Part model, mm, in its own coordinate system. Coordinates: 2 decimals unless noted, no trailing zeros. Write each loop counter-clockwise with the first axis right and the second up, starting at its lowest first coordinate (ties: lowest second). Pieces come first, ordered by that corner, then holes. Notation, with made-up numbers: (-40, 41.25) -> (-25, 41.25) arc R11 cw to (-25, 57.25) -> close; hole circle Ø4 at (59, -39). An arc over 180 degrees is marked (long way). One line per question, with ' | ' between items. Start each with the question number.
Item 1: Saw through at D-D (x = 0). List the corners of the cut face in (y, z), and give its area (3 significant figures).
Item 2: Two-plate mould, pull along Y, no slides. Class faces 1 (the cylindrical face through (-1.5, -4.5, -3.5)), 2 (the flat face through (-2, 0, -6)), 3 (the cylindrical face through (1.5, -4.5, -3.5)), 4 (the cylindrical face through (0.028, -5.158, -3.955)): pulls with the +Y half, pulls with the -Y half, needs draft (parallel to the pull), parting line crosses it, or undercut.
Item 3: Pin check, flat tips, straight feed: pin 1 (2 mm diameter, centred on x = 1.5, z = -3, fed in from -Y); pin 2 (3 mm diameter, centred on y = 0, z = 0, fed in from +X); pin 3 (2 mm diameter, centred on x = 1.5, y = -4, fed in from +Z); pin 4 (1 mm diameter, centred on x = -1.5, y = 3, fed in from +Z). Stop position of each tip, or through.
Item 4: Probe probe 1 along Z at (x, y) = (-1.65, 0); probe 2 along Z at (x, y) = (0.2, 0); probe 3 along Y at (x, z) = (1.45, -1.25). List the from-to ranges inside material, lowest first. Write a range as [from, to].
Item 5: Saw through at A-A (z = 0). List the corners of the cut face in (x, y).
Item 6: Saw through at C-C (x = 1.4). List the corners of the cut face in (y, z).
from build123d import *


with BuildPart() as part:
    # Esquisse1 → Révolution1 (revolve)
    with BuildSketch(Plane.XY):
        with BuildLine():
            Line((-2, 6.5), (2, 6.5))
            Line((2, 6.5), (2, 5.7))
            Line((2, 5.7), (1.058300524, 5.7))
            ThreePointArc((1.058300524, 5.7), (1.6, 4.5), (1.058300524, 3.3))
            Line((1.058300524, 3.3), (2, 3.3))
            Line((2, 3.3), (2, 2.5))
            Line((2, 2.5), (-2, 2.5))
            Line((-2, 2.5), (-2, 3.3))
            Line((-2, 3.3), (-1.058300524, 3.3))
            ThreePointArc((-1.058300524, 3.3), (-1.6, 4.5), (-1.058300524, 5.7))
            Line((-1.058300524, 5.7), (-2, 5.7))
            Line((-2, 5.7), (-2, 6.5))
        make_face()
    revolve(axis=Axis((-3.50151098, 0, 0), (1, 0, 0)))


solid = part.part
From the geometry:
1) outline: circle Ø13 at (0, 0); hole circle Ø5 at (0, 0) | area: 113 mm2
2) face 1: undercut | face 2: needs draft | face 3: undercut | face 4: parting line crosses it
3) pin 1: y = -6.18 | pin 2: through | pin 3: z = 5.77 | pin 4: z = 6
4) probe 1: [-6.5, -5.7], [-3.3, -2.5], [2.5, 3.3], [5.7, 6.5] | probe 2: [-6.5, -2.5], [2.5, 6.5] | probe 3: [-6.38, -5.56], [-5.02, -3.61], [-3.05, -2.17], [2.17, 3.05], [3.61, 5.02], [5.56, 6.38]
5) outline: (-2, -6.5) -> (2, -6.5) -> (2, -5.7) -> (1.06, -5.7) arc R1.6 ccw to (1.06, -3.3) -> (2, -3.3) -> (2, -2.5) -> (-2, -2.5) -> (-2, -3.3) -> (-1.06, -3.3) arc R1.6 ccw to (-1.06, -5.7) -> (-2, -5.7) -> close; (-2, 2.5) -> (2, 2.5) -> (2, 3.3) -> (1.06, 3.3) arc R1.6 ccw to (1.06, 5.7) -> (2, 5.7) -> (2, 6.5) -> (-2, 6.5) -> (-2, 5.7) -> (-1.06, 5.7) arc R1.6 ccw to (-1.06, 3.3) -> (-2, 3.3) -> close
6) outline: circle Ø13 at (0, 0); circle Ø10.55 at (0, 0); circle Ø6.6 at (0, 0); hole circle Ø11.4 at (0, 0); hole circle Ø7.45 at (0, 0); hole circle Ø5 at (0, 0)
